```python
from build123d import *

# Parameters (mm, degrees)
SKETCH1_R           = 75
BOSS_EXTRUDE3_DEPTH = 2
SKETCH2_R           = 1.5
CUT_EXTRUDE1_DEPTH  = 2
CIRPATTERN2_COUNT   = 8
SKETCH3_R           = 1.5
BOSS_EXTRUDE4_DEPTH = 2
SKETCH4_R           = 1.264823641
CUT_EXTRUDE2_DEPTH  = 10


with BuildPart() as part:
    # Sketch1 → Boss-Extrude3 (new body)
    with BuildSketch(Plane.XY):
        with Locations((6.9, 0)):
            Circle(SKETCH1_R)
        with BuildLine():
            Line((9.3, 1.8), (9.3, -1.8))
            ThreePointArc((9.3, -1.8), (3.9, 0), (9.3, 1.8))
        make_face(mode=Mode.SUBTRACT)
    extrude(amount=BOSS_EXTRUDE3_DEPTH)

    # Sketch2 → Cut-Extrude1 (cut)
    with BuildSketch(Plane.XY.offset(2)):
        with Locations((75.9, 0)):
            Circle(SKETCH2_R)
        with Locations((70.9, -7.5)):
            Circle(SKETCH2_R)
        with Locations((70.9, 7.5)):
            Circle(SKETCH2_R)
    cut_extrude1 = extrude(amount=-CUT_EXTRUDE1_DEPTH, mode=Mode.SUBTRACT)

    # CirPattern2: Cut-Extrude1 ×8 about axis
    cirpattern2_axis = Axis((6.9, 0, 0), (0, 0, 1))
    for i in range(1, CIRPATTERN2_COUNT):
        add(cut_extrude1.rotate(cirpattern2_axis, i * 360 / CIRPATTERN2_COUNT), mode=Mode.SUBTRACT)

    # Sketch3 → Boss-Extrude4 (add)
    with BuildSketch(Plane(origin=(0, 0, 0), x_dir=(-1, 0, 0), z_dir=(0, 0, -1))):
        with BuildLine():
            Line((-9.3, -1.8), (-9.3, 1.8))
            ThreePointArc((-9.3, 1.8), (-3.9, 0), (-9.3, -1.8))
        make_face()
        with Locations((-6.9, 0)):
            Circle(SKETCH3_R, mode=Mode.SUBTRACT)
    extrude(amount=-BOSS_EXTRUDE4_DEPTH)

    # Sketch4 → Cut-Extrude2 (cut)
    with BuildSketch(Plane.XY.offset(2)):
        with Locations((13.868293577, 4.129513848)):
            Circle(SKETCH4_R)
        with Locations((-0.068293577, -4.129513848)):
            Circle(SKETCH4_R)
    extrude(amount=-CUT_EXTRUDE2_DEPTH, mode=Mode.SUBTRACT)


solid = part.part
```
Read the model definition and answer for the solid it produces. Units are mm, in the model's axes. Coordinates: 2 decimals unless noted, no trailing zeros. Write each loop counter-clockwise with the first axis right and the second up, starting at its lowest first coordinate (ties: lowest second). Pieces come first, ordered by that corner, then holes. Notation, with made-up numbers: (50.5, 28.25) - (89.5, 28.25) arc R26 cw to (89.5, 51.25) - close; hole circle Ø10 at (-18, -4.5). An arc over 180 degrees is marked (long way). Answer as a JSON object with one key per item and string values. Group by question number.
1. A cutting plane is placed at A-A (z = 1). Give the number of separate pieces and of enclosed holes in the cut face, plus the area to 3 significant figures.
2. A cutting plane is placed at B-B (x = 29). Determine the outline of the cut face in (y, z), plus the area to 3 significant figures.
3. Consider L1, parallel to X at y = -51.5, z = 0.6; L2, parallel to X at y = -65, z = 0.2; L3, parallel to Y at x = 55.5, z = 0.7. Determine where each line is inside the solid, lowest interval first. Write a range as [from, to].
4. A cutting plane is placed at C-C (y = -34.5). Determine the outline of the cut face in (x, z), plus the area to 3 significant figures.
5. This flat-tipped pin is pushed along its axis until it touches: P1, Ø1, axis at y = 57, z = 1, coming from the -X side. Where does it stop, or does it pass through?
Worked out:
{
 "1": {"separate pieces": "1", "enclosed holes": "27", "area": "17,500 mm²"},
 "2": {"outline": "(-71.67, 0) - (71.67, 0) - (71.67, 2) - (-71.67, 2) - close", "area": "287 mm²"},
 "3": {"L1": "x = [-47.62, -34.22], [-31.88, 45.68], [48.02, 61.42]", "L2": "x = [-30.52, -1.72], [0.52, 13.28], [15.52, 44.32]", "L3": "y = [-57.12, -50.28], [-47.3, 47.3], [50.28, 57.12]"},
 "4": {"outline": "(-59.69, 0) - (73.49, 0) - (73.49, 2) - (-59.69, 2) - close", "area": "266 mm²"},
 "5": {"P1": "stops at x = -42.42"}
}
